```python
from build123d import *

# Parameters (mm, degrees)
SKETCH_1_R      = 1.75
EXTRUDE_1_DEPTH = 3
FILLET_1_R      = 5
MM_1_D          = 4


with BuildPart() as part:
    # 草图1 → 凸台-拉伸1 (new body)
    with BuildSketch(Plane.XY):
        with BuildLine():
            Line((-29.416994756, 204), (29.416994756, 204))
            Line((29.416994756, 204), (40, 192))
            Line((40, 192), (40, 182))
            Line((40, 182), (59.356157589, 179))
            ThreePointArc((59.356157589, 179), (61.5, 172), (59.356157589, 165))
            Line((59.356157589, 165), (40, 162))
            Line((40, 162), (40, 142))
            Line((40, 142), (55.5, 90))
            Line((55.5, 90), (55.5, 0))
            Line((55.5, 0), (-55.5, 0))
            Line((-55.5, 0), (-55.5, 90))
            Line((-55.5, 90), (-40, 142))
            Line((-40, 142), (-40, 162))
            Line((-40, 162), (-59.356157589, 165))
            ThreePointArc((-59.356157589, 165), (-61.5, 172), (-59.356157589, 179))
            Line((-59.356157589, 179), (-40, 182))
            Line((-40, 182), (-40, 192))
            Line((-40, 192), (-29.416994756, 204))
        make_face()
        with Locations((-49, 172)):
            Circle(SKETCH_1_R, mode=Mode.SUBTRACT)
        with Locations((49, 172)):
            Circle(SKETCH_1_R, mode=Mode.SUBTRACT)
        with Locations((39, 172)):
            Circle(SKETCH_1_R, mode=Mode.SUBTRACT)
        with Locations((-39, 172)):
            Circle(SKETCH_1_R, mode=Mode.SUBTRACT)
    extrude(amount=EXTRUDE_1_DEPTH)

    # 圆角1
    fillet_1_edges = [part.edges().sort_by_distance(p)[0] for p in [
        (55.5, 0, 1.5),
        (-55.5, 0, 1.5),
    ]]
    fillet(fillet_1_edges, radius=FILLET_1_R)

    # 大小mm 暗销孔1 (through all)
    with Locations(Plane(origin=(0, 0, 0), x_dir=(-1, 0, 0), z_dir=(0, 0, -1))):
        with Locations((-32.25, 160), (32.25, 160), (44, 63), (-44, 63)):
            Hole(MM_1_D / 2)


solid = part.part
```
The model under review builds one solid part; all positions refer to its coordinate system, in mm. A direction names the side the tool comes from. Give positions to 0.01 mm unless a question says otherwise; leave off trailing zeros. Write each loop counter-clockwise with the first axis right and the second up, starting at its lowest first coordinate (ties: lowest second). Pieces come first, ordered by that corner, then holes. Notation, with made-up numbers: (63.25, 30.5) - (120.25, 30.5) arc R31 cw to (120.25, 58.5) - close; hole circle Ø1 at (-34, 84). An arc over 180 degrees is marked (long way). Answer in a Markdown table with one row per item. Add a question column.
1. We need section A-A on z = 0.9. State how many separate pieces and enclosed holes the cut face has, then the cut area to 3 significant figures.
2. Insertion check: P1, Ø5.5, axis at x = -49, y = 172, coming from the -Z side; P2, Ø1.5, axis at y = 153, z = 1, coming from the -X side; P3, Ø1, axis at y = 67.5, z = 2, coming from the +X side. Each pin has a flat end and moves straight along its axis. Give the tip position at first contact, or say it passes through.
3. We need section C-C on x = 32.25. Write out the cut boundary in (y, z).
4. Tool access review of faces 4 (the flat face through (-47.858, 115.636, 1.479)), 5 (the flat face through (47.642, 116.364, 1.479)), 6 (the flat face through (-34.78, 197.92, 1.48)): name each direction out of +Z, -Z, +X, -X, +Y, -Y from which nothing blocks a thin tool from reaching the whole face with its end or side.
5. We need section B-B on x = -44. Write out the cut boundary in (y, z), then the cut area to 3 significant figures.
6. We need section D-D on y = 151. Write out the cut boundary in (x, z).
7. Wall thickness on line 1 along X through (y, z) = (172, 1.15); line 2 along X through (y, z) = (160, 2.15); line 3 along X through (y, z) = (68, 1.8): over which ranges is each line inside the solid? List them lowest first. Write a range as [from, to].
8. Draft analysis for pull direction Y (two halves, no side actions). For faces 1 (the flat face through (1, 103, 3)), 2 (the cylindrical face through (45.075, 64.686, 1.521)), 3 (the flat face through (34.634, 198.084, 1.479)), state which applies: +Y half, -Y half, draft (parallel to the pull), parting line (faces both ways), or undercut.
Ans:
| question | item | result |
|---|---|---|
| 1 | separate pieces | 1 |
| 1 | enclosed holes | 8 |
| 1 | area | 20,400 mm^2 |
| 2 | P1 | stops at z = 0 |
| 2 | P2 | stops at x = -40 |
| 2 | P3 | stops at x = 55.5 |
| 3 | outline | (0, 0) - (158, 0) - (158, 3) - (0, 3) - close; (162, 0) - (200.79, 0) - (200.79, 3) - (162, 3) - close |
| 4 | face 4 | +Z, -Z, -X |
| 4 | face 5 | +Z, -Z, +X |
| 4 | face 6 | +Z, -Z, -X, +Y |
| 5 | outline | (0, 0) - (61, 0) - (61, 3) - (0, 3) - close; (65, 0) - (128.58, 0) - (128.58, 3) - (65, 3) - close; (162.62, 0) - (181.38, 0) - (181.38, 3) - (162.62, 3) - close |
| 5 | area | 430 mm^2 |
| 6 | outline | (-40, 0) - (40, 0) - (40, 3) - (-40, 3) - close |
| 7 | line 1 | x = [-61.5, -50.75], [-47.25, -40.75], [-37.25, 37.25], [40.75, 47.25], [50.75, 61.5] |
| 7 | line 2 | x = [-40, -34.25], [-30.25, 30.25], [34.25, 40] |
| 7 | line 3 | x = [-55.5, 55.5] |
| 8 | face 1 | draft |
| 8 | face 2 | undercut |
| 8 | face 3 | +Y half |
